Can you work these out from the model? Positions are in its coordinate system, mm. A direction names the side the tool comes from. Give positions to 0.01 mm unless a question says otherwise; leave off trailing zeros. Loops run counter-clockwise (first coordinate to the right, second up) from the corner with the lowest first, then second, coordinate; pieces in that order, holes last. Notation, with made-up numbers: (80.25, 39.25) - (137.25, 39.25) arc R20 cw to (137.25, 53.25) - close; hole circle Ø8 at (-12.75, 71.25). An arc over 180 degrees is marked (long way). Answer as a JSON object with one key per item and string values.
```python
from build123d import *

# Parameters (mm, degrees)
F0_W        = 127
F0_H        = 88.9
F1_DEPTH    = 38.1
F2_T        = -2.54
F3_T1_DEPTH = 231.5131966309
F4_R        = 5.08
F5_R        = 6.333111045
F6_DEPTH    = 25.4


# Not quite as in the source:
# - a fillet or chamfer that OpenCascade refuses, or shapes differently, is made with other operations: its cross-section is extruded or revolved along the edge and cut away or added


with BuildPart() as f1:
    # F0 (on Front) → F1 (new body)
    with BuildSketch(Plane.XZ):
        Rectangle(F0_W, F0_H)
    extrude(amount=-F1_DEPTH)

    # F2
    f2_openings = [f1.faces().sort_by_distance(p)[0] for p in [
        (0, 19.05, 44.45),
    ]]
    offset(amount=F2_T, openings=f2_openings)

    # F3: chamfer of 20.32 on 1 edges, made by hand

    # F3_s2 → F3_t1 (cut)
    with BuildSketch(Plane.YZ.offset(-115.7565983155)):
        Polygon((0, 24.13), (20.32, 44.45), (0, 44.45), align=None)
    extrude(amount=F3_T1_DEPTH, mode=Mode.SUBTRACT)

    # F4
    f4_edges = [f1.edges().sort_by_distance(p)[0] for p in [
        (-63.5, 10.16, 34.29),
        (63.5, 10.16, 34.29),
        (0, 0, 24.13),
    ]]
    fillet(f4_edges, radius=F4_R)

    # F5 (on face) → F6 (cut)
    with BuildSketch(Plane(origin=(0, 38.1, 0), x_dir=(-1, 0, 0), z_dir=(0, 1, 0))):
        with Locations((-48.4922043979, 28.5164732486)):
            Circle(F5_R)
        with Locations((48.4922043979, 28.5164732486)):
            Circle(F5_R)
    extrude(amount=-F6_DEPTH, mode=Mode.SUBTRACT)


solid = f1.part
```
1) Imagine slicing it at C-C on y = 30.5. Write out the boundary of the cut face in (x, z).
Check sheet entries:
{"outline": "(-63.5, -44.45) - (63.5, -44.45) - (63.5, 44.45) - (60.96, 44.45) - (60.96, -41.91) - (-60.96, -41.91) - (-60.96, 44.45) - (-63.5, 44.45) - close"}
2) Imagine slicing it at D-D on x = 53.5. Write out the boundary of the cut face in (y, z).
Check sheet entries:
{"outline": "(0, -44.45) - (38.1, -44.45) - (38.1, 24.64) - (35.56, 24.64) - (35.56, -41.91) - (2.54, -41.91) - (2.54, 26.67) - (1.49, 25.62) arc R5.08 ccw to (0, 22.03) - close; (35.56, 32.39) - (38.1, 32.39) - (38.1, 44.45) - (35.56, 44.45) - close"}
3) Which directions (+Z, -Z, +X, -X, +Y, -Y) give clear straight access to the entire face, cutting with the end or side of a thin tool? Please do faces 1 (the cylindrical face through (42.45, 36.85, 30.42)), 2 (the flat face through (-1, 19, -41.91)), 3 (the flat face through (-10, 36, 44.45)).
Check sheet entries:
{"face 1": "+Y", "face 2": "+Z", "face 3": "+Z, +X, -X, +Y, -Y"}
4) I'm going to push flat-ended pins straight in: P1, Ø1, axis at x = 50, y = 31, coming from the +Z side; P2, Ø6, axis at x = 5, z = 33.5, coming from the -Y side. Where does each tip first touch, or does it pass through?
Check sheet entries:
{"P1": "z = -41.91", "P2": "y = 35.56"}
5) Imagine slicing it at A-A on z = 8.5. Write out the boundary of the cut face in (x, y), and give its area (3 significant figures).
Check sheet entries:
{"outline": "(-63.5, 0) - (63.5, 0) - (63.5, 38.1) - (-63.5, 38.1) - close; hole (-60.96, 2.54) - (60.96, 2.54) - (60.96, 35.56) - (-60.96, 35.56) - close", "area": "813 mm2"}
6) If we mould it in two halves opening along Y, with no side actions, what happens to faces 4 (the flat face through (-1, 0, -11)), 5 (the flat face through (-60.96, 19, 1)), 6 (the cylindrical face through (-54.533, 36.848, 30.419)), 7 (the flat face through (-1, 38.1, 1))? For each: released by +Y, released by -Y, zero draft, split by the parting line, or undercut.
Check sheet entries:
{"face 4": "released by -Y", "face 5": "undercut", "face 6": "zero draft", "face 7": "released by +Y"}
7) I need wall thicknesses on L1, parallel to X at y = 19, z = 9; L2, parallel to Y at x = -23, z = 10; L3, parallel to Z at x = 41, y = 13. Which ranges of each line are inside material? Lowest first, please.
Check sheet entries:
{"L1": "-63.5 to -60.96, 60.96 to 63.5", "L2": "0 to 2.54, 35.56 to 38.1", "L3": "-44.45 to -41.91"}
8) Imagine slicing it at B-B on x = -27.5. Write out the boundary of the cut face in (y, z).
Check sheet entries:
{"outline": "(0, -44.45) - (38.1, -44.45) - (38.1, 44.45) - (35.56, 44.45) - (35.56, -41.91) - (2.54, -41.91) - (2.54, 26.67) - (1.49, 25.62) arc R5.08 ccw to (0, 22.03) - close"}
